from build123d import *

# Parameters (mm, degrees)
SK_MAIN_EXTRUSION_R  = 3.4
MAIN_EXTRUSION_DEPTH = 25


with BuildPart() as part:
    # Sk Main Extrusion → Main Extrusion (new body)
    with BuildSketch(Plane.XY):
        with BuildLine():
            Line((-4.190076845, 16.671180212), (-5.222054351, 19.506515107))
            ThreePointArc((-5.222054351, 19.506515107), (-5.496641489, 19.864364033), (-5.926823816, 20))
            Line((-5.926823816, 20), (-18.5, 20))
            ThreePointArc((-18.5, 20), (-19.560660172, 19.560660172), (-20, 18.5))
            Line((-20, 18.5), (-20, -18.5))
            ThreePointArc((-20, -18.5), (-19.560660172, -19.560660172), (-18.5, -20))
            Line((-18.5, -20), (-5.926823816, -20))
            ThreePointArc((-5.926823816, -20), (-5.496641489, -19.864364033), (-5.222054351, -19.506515107))
            Line((-5.222054351, -19.506515107), (-4.190076845, -16.671180212))
            ThreePointArc((-4.190076845, -16.671180212), (-4.175951325, -16.563886241), (-4.208493649, -16.460675177))
            Line((-4.208493649, -16.460675177), (-4.987558066, -15.111296024))
            Line((-4.987558066, -15.111296024), (-5.718509166, -14.845251581))
            Line((-5.718509166, -14.845251581), (-8.396186179, -15.81984631))
            ThreePointArc((-8.396186179, -15.81984631), (-8.811074612, -15.786489799), (-9.056960151, -15.450654467))
            ThreePointArc((-9.056960151, -15.450654467), (-8.933433013, -12.665882372), (-7.504160339, -10.272684887))
            Line((-7.504160339, -10.272684887), (-6.540737726, -9.309262274))
            ThreePointArc((-6.540737726, -9.309262274), (0, -6.6), (6.540737726, -9.309262274))
            Line((6.540737726, -9.309262274), (7.504160339, -10.272684887))
            ThreePointArc((7.504160339, -10.272684887), (8.933433013, -12.665882372), (9.056960151, -15.450654467))
            ThreePointArc((9.056960151, -15.450654467), (8.811074612, -15.786489799), (8.396186179, -15.81984631))
            Line((8.396186179, -15.81984631), (5.718509166, -14.845251581))
            Line((5.718509166, -14.845251581), (4.987558066, -15.111296024))
            Line((4.987558066, -15.111296024), (4.208493649, -16.460675177))
            ThreePointArc((4.208493649, -16.460675177), (4.175951325, -16.563886241), (4.190076845, -16.671180212))
            Line((4.190076845, -16.671180212), (5.222054351, -19.506515107))
            ThreePointArc((5.222054351, -19.506515107), (5.496641489, -19.864364033), (5.926823816, -20))
            Line((5.926823816, -20), (18.5, -20))
            ThreePointArc((18.5, -20), (19.560660172, -19.560660172), (20, -18.5))
            Line((20, -18.5), (20, 18.5))
            ThreePointArc((20, 18.5), (19.560660172, 19.560660172), (18.5, 20))
            Line((18.5, 20), (5.926823816, 20))
            ThreePointArc((5.926823816, 20), (5.496641489, 19.864364033), (5.222054351, 19.506515107))
            Line((5.222054351, 19.506515107), (4.190076845, 16.671180212))
            ThreePointArc((4.190076845, 16.671180212), (4.175951325, 16.563886241), (4.208493649, 16.460675177))
            Line((4.208493649, 16.460675177), (4.987558066, 15.111296024))
            Line((4.987558066, 15.111296024), (5.718509166, 14.845251581))
            Line((5.718509166, 14.845251581), (8.396186179, 15.81984631))
            ThreePointArc((8.396186179, 15.81984631), (8.811074612, 15.786489799), (9.056960151, 15.450654467))
            ThreePointArc((9.056960151, 15.450654467), (8.933433013, 12.665882372), (7.504160339, 10.272684887))
            Line((7.504160339, 10.272684887), (6.540737726, 9.309262274))
            ThreePointArc((6.540737726, 9.309262274), (0, 6.6), (-6.540737726, 9.309262274))
            Line((-6.540737726, 9.309262274), (-7.504160339, 10.272684887))
            ThreePointArc((-7.504160339, 10.272684887), (-8.933433013, 12.665882372), (-9.056960151, 15.450654467))
            ThreePointArc((-9.056960151, 15.450654467), (-8.811074612, 15.786489799), (-8.396186179, 15.81984631))
            Line((-8.396186179, 15.81984631), (-5.718509166, 14.845251581))
            Line((-5.718509166, 14.845251581), (-4.987558066, 15.111296024))
            Line((-4.987558066, 15.111296024), (-4.208493649, 16.460675177))
            ThreePointArc((-4.208493649, 16.460675177), (-4.175951325, 16.563886241), (-4.190076845, 16.671180212))
        make_face()
        Circle(SK_MAIN_EXTRUSION_R, mode=Mode.SUBTRACT)
        with BuildLine():
            Line((-8.308504679, 7.441495321), (-9.444282589, 8.577273231))
            ThreePointArc((-9.444282589, 8.577273231), (-11.611987193, 12.430514315), (-11.464011904, 16.849169473))
            ThreePointArc((-11.464011904, 16.849169473), (-11.537349181, 17.295452819), (-11.940719521, 17.5))
            Line((-11.940719521, 17.5), (-17, 17.5))
            ThreePointArc((-17, 17.5), (-17.353553391, 17.353553391), (-17.5, 17))
            Line((-17.5, 17), (-17.5, 1.75))
            ThreePointArc((-17.5, 1.75), (-17.353553391, 1.396446609), (-17, 1.25))
            Line((-17, 1.25), (-6.156094541, 1.25))
            ThreePointArc((-6.156094541, 1.25), (-5.854730455, 1.351026708), (-5.675149655, 1.61328125))
            ThreePointArc((-5.675149655, 1.61328125), (-5.51245547, 2.10305366), (-5.307583096, 2.576734694))
            ThreePointArc((-5.307583096, 2.576734694), (-5.153883821, 4.359333373), (-6.230846881, 5.788120301))
            ThreePointArc((-6.230846881, 5.788120301), (-7.316529108, 6.555931161), (-8.308504679, 7.441495321))
        make_face(mode=Mode.SUBTRACT)
        with BuildLine():
            Line((-17.5, -1.75), (-17.5, -17))
            ThreePointArc((-17.5, -17), (-17.353553391, -17.353553391), (-17, -17.5))
            Line((-17, -17.5), (-11.940719521, -17.5))
            ThreePointArc((-11.940719521, -17.5), (-11.537349181, -17.295452819), (-11.464011904, -16.849169473))
            ThreePointArc((-11.464011904, -16.849169473), (-11.611987193, -12.430514315), (-9.444282589, -8.577273231))
            Line((-9.444282589, -8.577273231), (-8.308504679, -7.441495321))
            ThreePointArc((-8.308504679, -7.441495321), (-7.316529108, -6.555931161), (-6.230846881, -5.788120301))
            ThreePointArc((-6.230846881, -5.788120301), (-5.153883821, -4.359333373), (-5.307583096, -2.576734694))
            ThreePointArc((-5.307583096, -2.576734694), (-5.51245547, -2.10305366), (-5.675149655, -1.61328125))
            ThreePointArc((-5.675149655, -1.61328125), (-5.854730455, -1.351026708), (-6.156094541, -1.25))
            Line((-6.156094541, -1.25), (-17, -1.25))
            ThreePointArc((-17, -1.25), (-17.353553391, -1.396446609), (-17.5, -1.75))
        make_face(mode=Mode.SUBTRACT)
        with BuildLine():
            Line((9.444282589, 8.577273231), (8.308504679, 7.441495321))
            ThreePointArc((8.308504679, 7.441495321), (7.316529108, 6.555931161), (6.230846881, 5.788120301))
            ThreePointArc((6.230846881, 5.788120301), (5.153883821, 4.359333373), (5.307583096, 2.576734694))
            ThreePointArc((5.307583096, 2.576734694), (5.51245547, 2.10305366), (5.675149655, 1.61328125))
            ThreePointArc((5.675149655, 1.61328125), (5.854730455, 1.351026708), (6.156094541, 1.25))
            Line((6.156094541, 1.25), (17, 1.25))
            ThreePointArc((17, 1.25), (17.353553391, 1.396446609), (17.5, 1.75))
            Line((17.5, 1.75), (17.5, 17))
            ThreePointArc((17.5, 17), (17.353553391, 17.353553391), (17, 17.5))
            Line((17, 17.5), (11.940719521, 17.5))
            ThreePointArc((11.940719521, 17.5), (11.537349181, 17.295452819), (11.464011904, 16.849169473))
            ThreePointArc((11.464011904, 16.849169473), (11.611987193, 12.430514315), (9.444282589, 8.577273231))
        make_face(mode=Mode.SUBTRACT)
        with BuildLine():
            Line((8.308504679, -7.441495321), (9.444282589, -8.577273231))
            ThreePointArc((9.444282589, -8.577273231), (11.611987193, -12.430514315), (11.464011904, -16.849169473))
            ThreePointArc((11.464011904, -16.849169473), (11.537349181, -17.295452819), (11.940719521, -17.5))
            Line((11.940719521, -17.5), (17, -17.5))
            ThreePointArc((17, -17.5), (17.353553391, -17.353553391), (17.5, -17))
            Line((17.5, -17), (17.5, -1.75))
            ThreePointArc((17.5, -1.75), (17.353553391, -1.396446609), (17, -1.25))
            Line((17, -1.25), (6.156094541, -1.25))
            ThreePointArc((6.156094541, -1.25), (5.854730455, -1.351026708), (5.675149655, -1.61328125))
            ThreePointArc((5.675149655, -1.61328125), (5.51245547, -2.10305366), (5.307583096, -2.576734694))
            ThreePointArc((5.307583096, -2.576734694), (5.153883821, -4.359333373), (6.230846881, -5.788120301))
            ThreePointArc((6.230846881, -5.788120301), (7.316529108, -6.555931161), (8.308504679, -7.441495321))
        make_face(mode=Mode.SUBTRACT)
    extrude(amount=-MAIN_EXTRUSION_DEPTH)


solid = part.part
Work out the finished part from the listing and answer in its coordinate system (mm). A direction names the side the tool comes from. Coordinates: 2 decimals unless noted, no trailing zeros. Loops run counter-clockwise (first coordinate to the right, second up) from the corner with the lowest first, then second, coordinate; pieces in that order, holes last. Notation, with made-up numbers: M -38.75,0 L -8.75,0 A21 ccw -8.75,37 Z; hole C 12,18 d3. An arc over 180 degrees is marked long. Answer in a Markdown table with one row per item. Add a question column.
1. Find section D-D, the plane y = -14. Write down the section's boundary in (x, z).
2. Find section C-C, the plane x = 2.5. Write down the section's boundary in (y, z).
3. Consider L1, parallel to Y at x = -16.5, z = -11.75; L2, parallel to Y at x = 0, z = -15.5. Determine where each line is inside the solid, lowest interval first.
4. Find section A-A, the plane x = 13. Write down the section's boundary in (y, z), then the cut area to 4 significant figures.
5. The mould has two halves that part along Y. Classify faces 3 (the flat face through (20, 0, -12)), 4 (the cylindrical face through (-5.147, 4.335, -12.325)), 5 (the flat face through (4.713, 18.109, -12.325)): pulls with the +Y half, pulls with the -Y half, needs draft (parallel to the pull), parting line crosses it, or undercut.
6. A tool of negligible diameter and unlimited length cuts with its end or side. For faces 1 (the flat face through (-12, 1.25, -12)), 2 (the flat face through (-4.7, 18.07, -12.32)), from which of +Z, -Z, +X, -X, +Y, -Y can it reach the whole face along a straight path? Write none if from no direction.
7. A flat-ended cylindrical pin translates along its axis: P1, Ø8, axis at x = 1.5, z = -22, coming from the +Y side. Find the tip coordinate at first contact, or state that the pin passes through.
8. Find section B-B, the plane y = 0. Write down the section's boundary in (x, z), then the cut area to 3 significant figures.
Reported:
| question | item | result |
|---|---|---|
| 1 | outline | M -20,-25 L -17.5,-25 L -17.5,0 L -20,0 Z; M -11.84,-25 L -9.17,-25 L -9.17,0 L -11.84,0 Z; M 9.17,-25 L 11.84,-25 L 11.84,0 L 9.17,0 Z; M 17.5,-25 L 20,-25 L 20,0 L 17.5,0 Z |
| 2 | outline | M -6.94,-25 L -2.3,-25 L -2.3,0 L -6.94,0 Z; M 2.3,-25 L 6.94,-25 L 6.94,0 L 2.3,0 Z |
| 3 | L1 | y = -20 to -17.5, -1.25 to 1.25, 17.5 to 20 |
| 3 | L2 | y = -6.6 to -3.4, 3.4 to 6.6 |
| 4 | outline | M -20,-25 L -17.5,-25 L -17.5,0 L -20,0 Z; M -1.25,-25 L 1.25,-25 L 1.25,0 L -1.25,0 Z; M 17.5,-25 L 20,-25 L 20,0 L 17.5,0 Z |
| 4 | area | 187.5 mm^2 |
| 5 | face 3 | needs draft |
| 5 | face 4 | undercut |
| 5 | face 5 | pulls with the +Y half |
| 6 | face 1 | +Z, -Z |
| 6 | face 2 | +Z, -Z, +Y |
| 7 | P1 | stops at y = 19.87 |
| 8 | outline | M -20,-25 L -3.4,-25 L -3.4,0 L -20,0 Z; M 3.4,-25 L 20,-25 L 20,0 L 3.4,0 Z |
| 8 | area | 830 mm^2 |
